Here's how the part is built. I have some questions about the finished solid (model axes, mm). Face numbers are marked on the shaded views. A direction names the side the tool comes from. Coordinates: 2 decimals unless noted, no trailing zeros. Write each loop counter-clockwise with the first axis right and the second up, starting at its lowest first coordinate (ties: lowest second). Pieces come first, ordered by that corner, then holes. Notation, with made-up numbers: (36.5, 14) -> (44.5, 14) arc R21 ccw to (44.5, 47) -> close; hole circle Ø7 at (76.5, 68.5). An arc over 180 degrees is marked (long way). Put each result on its own line as item: value. Start each with the question number.
Item 1: For pin 1 (6 mm diameter, centred on y = 15.5, z = 22.5, fed in from -X); pin 2 (12 mm diameter, centred on y = -4.5, z = 31, fed in from -X); pin 3 (14 mm diameter, centred on y = -0.5, z = 26.5, fed in from +X), each with a flat end and sliding along its axis, tell me the tip position at first contact or that it passes through.
Item 2: I want a section at A-A, the plane x = -56.11. List the corners of the cut face in (y, z) for me (3 decimals).
Item 3: I want a section at C-C, the plane x = 7.5. List the corners of the cut face in (y, z) for me, then the cut area to 3 significant figures.
Item 4: I need wall thicknesses on line 1 (X direction, y = -2, z = 2) (3 decimals); line 2 (X direction, y = -4.5, z = 34); line 3 (Y direction, x = -32.5, z = 29.5). Which ranges of each line are inside material? Lowest first, please. Write a range as [from, to].
Item 5: If we mould it in two halves opening along X, with no side actions, what happens to the marked faces 1, 2, 3 and 4? For each: released by +X, released by -X, zero draft, split by the parting line, or undercut.
Item 6: I want a section at D-D, the plane y = 6. List the corners of the cut face in (x, z) for me, then the cut area to 3 significant figures.
Item 7: I want a section at B-B, the plane z = 13.5. List the corners of the cut face in (x, y) for me.
Item 8: On a 3-axis mill with a long thin cutter (end or side, diameter ignored), from which of +Z, -Z, +X, -X, +Y, -Y can I reach the whole of each face in a straight line? I mean the marked faces 5, 6 and 7. Say none if no direction works.
from build123d import *

# Parameters (mm, degrees)
F0_W           = 84.22
F0_H           = 33.42
F0_W_2         = 20
F0_H_2         = 4
F1_DEPTH       = 38.1
F0_H_3         = 37.42
F2_DEPTH       = 6
F4_D           = 6.35
F4_CSINK_D     = 12.7
F4_CSINK_ANGLE = 90
F6_DEPTH       = 25
F7_R           = 4


with BuildPart() as f1:
    # F0 (on Top) → F1 (new body)
    with BuildSketch(Plane.XY):
        Polygon((46.11, 16.71), (46.11, 20.71), (-46.11, 20.71), (-46.11, 16.71), (-46.11, -20.71), (46.11, -20.71), align=None)
        Rectangle(F0_W, F0_H, mode=Mode.SUBTRACT)
        with Locations((56.11, 18.71)):
            Rectangle(F0_W_2, F0_H_2)
        with Locations((-56.11, 18.71)):
            Rectangle(F0_W_2, F0_H_2)
    extrude(amount=F1_DEPTH)

    # F0 (on Top) → F2 (join)
    with BuildSketch(Plane.XY):
        with Locations((-56.11, -2)):
            Rectangle(F0_W_2, F0_H_3)
        with Locations((56.11, -2)):
            Rectangle(F0_W_2, F0_H_3)
        Rectangle(F0_W, F0_H)
    extrude(amount=F2_DEPTH)

    # F4 (through all)
    with Locations(Plane.XY.offset(6)):
        with Locations((-56.11, -2), (56.11, -2)):
            CounterSinkHole(F4_D / 2, F4_CSINK_D / 2, counter_sink_angle=F4_CSINK_ANGLE)

    # F5 (on face) → F6 (cut)
    with BuildSketch(Plane(origin=(0, 20.71, 0), x_dir=(-1, 0, 0), z_dir=(0, 1, 0))):
        Polygon((-66.11, 6), (-46.11, 38.1), (-66.11, 38.1), align=None)
        Polygon((66.11, 38.1), (46.11, 38.1), (66.11, 6), align=None)
    extrude(amount=-F6_DEPTH, mode=Mode.SUBTRACT)

    # F7
    f7_edges = [f1.edges().sort_by_distance(p)[0] for p in [
        (46.11, 16.71, 22.05),
        (-46.11, 16.71, 22.05),
        (-46.11, -2, 6),
        (-56.11, 16.71, 6),
        (46.11, -2, 6),
        (56.11, 16.71, 6),
    ]]
    fillet(f7_edges, radius=F7_R)


solid = f1.part
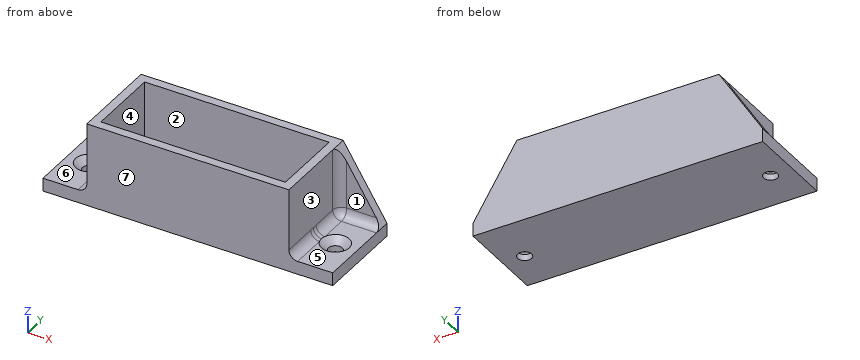
Calculated:
1. pin 1: stops at x = -57.54
1. pin 2: stops at x = -46.11
1. pin 3: stops at x = 46.11
2. outline: (-20.71, 0) -> (-5.175, 0) -> (-5.175, 2.825) -> (-8.35, 6) -> (-20.71, 6) -> close; (1.175, 0) -> (20.71, 0) -> (20.71, 22.05) -> (16.71, 22.05) -> (16.71, 10) arc R4 cw to (12.71, 6) -> (4.35, 6) -> (1.175, 2.825) -> close
3. outline: (-20.71, 0) -> (20.71, 0) -> (20.71, 38.1) -> (16.71, 38.1) -> (16.71, 6) -> (-16.71, 6) -> (-16.71, 38.1) -> (-20.71, 38.1) -> close
3. area: 505 mm2
4. line 1: x = [-66.11, -59.285], [-52.935, 52.935], [59.285, 66.11]
4. line 2: x = [-46.11, -42.11], [42.11, 46.11]
4. line 3: y = [-20.71, -16.71], [16.71, 20.71]
5. face 1: zero draft
5. face 2: undercut
5. face 3: released by +X
5. face 4: undercut
6. outline: (-66.11, 0) -> (66.11, 0) -> (66.11, 6) -> (50.11, 6) arc R4 cw to (46.11, 10) -> (46.11, 38.1) -> (42.11, 38.1) -> (42.11, 6) -> (-42.11, 6) -> (-42.11, 38.1) -> (-46.11, 38.1) -> (-46.11, 10) arc R4 cw to (-50.11, 6) -> (-66.11, 6) -> close
6. area: 1,060 mm2
7. outline: (-61.44, 16.71) -> (-50.11, 16.71) arc R4 cw to (-46.11, 12.71) -> (-46.11, -20.71) -> (46.11, -20.71) -> (46.11, 12.71) arc R4 cw to (50.11, 16.71) -> (61.44, 16.71) -> (61.44, 20.71) -> (-61.44, 20.71) -> close; hole (-42.11, -16.71) -> (42.11, -16.71) -> (42.11, 16.71) -> (-42.11, 16.71) -> close
8. face 5: +Z, +X, -Y
8. face 6: +Z, -X, -Y
8. face 7: +Z, -Z, +X, -X, -Y
